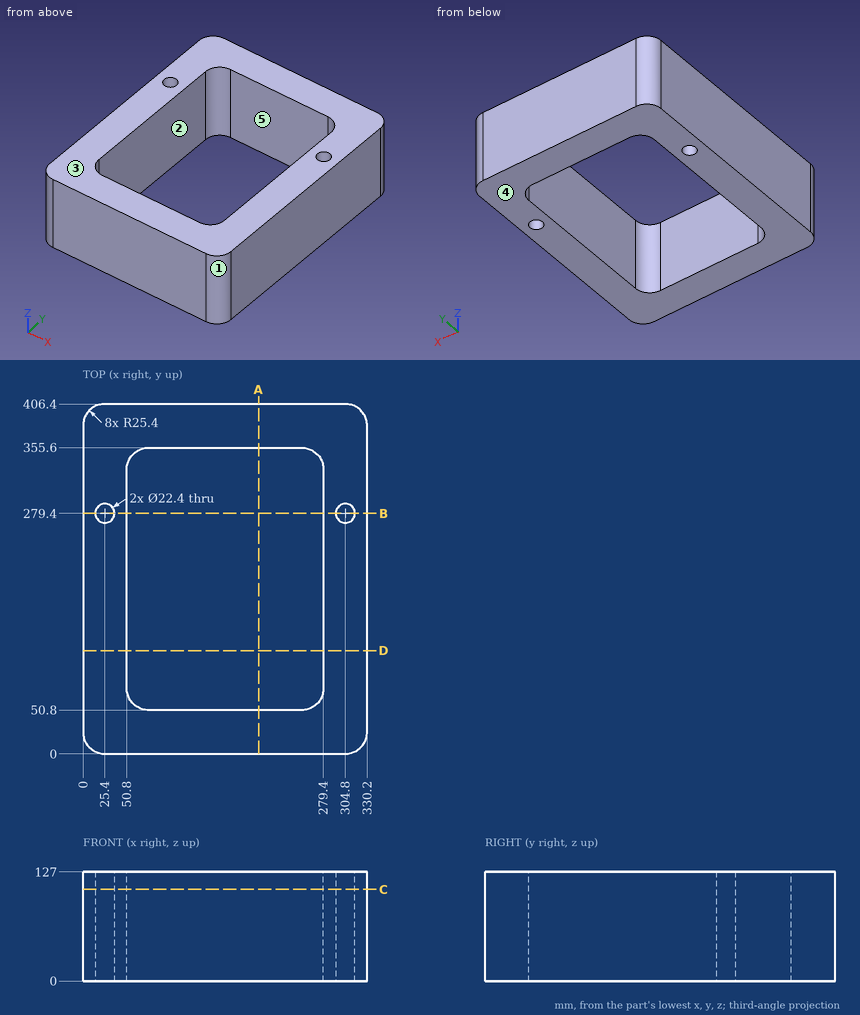
Geometry: see drawing. Coordinates: mm, zero at the bounding-box minimum. A direction names the side the tool comes from. Give positions to 0.01 mm unless a question says otherwise; leave off trailing zeros. Loops run counter-clockwise (first coordinate to the right, second up) from the corner with the lowest first, then second, coordinate; pieces in that order, holes last. Notation, with made-up numbers: (68.25, 50.25) -> (121.25, 50.25) arc R17 ccw to (121.25, 78.25) -> close; hole circle Ø9 at (81.25, -39). An arc over 180 degrees is marked (long way). Use one line per item in the form item = value.
Item 1: Section query D-D on y = 120. Output: boundary loops of the cut face in (x, z).
A:
outline = (0, 0) -> (50.8, 0) -> (50.8, 127) -> (0, 127) -> close; (279.4, 0) -> (330.2, 0) -> (330.2, 127) -> (279.4, 127) -> close
Item 2: Pin query (flat end, axial travel): P1, Ø2, axis at x = 222, z = 35, coming from the -Y side. Return the tip coordinate at first contact, or that it passes through.
A:
P1 = 0
Item 3: Access query for the marked faces 4 and 5. Directions: +Z, -Z, +X, -X, +Y, -Y. A direction counts if a zero-diameter tool reaches every point of the face in a straight line with its end or side. Return the directions, or none.
A:
face_4 = -Z, +X, -X, +Y, -Y
face_5 = +Z, -Z
Item 4: Section query B-B on y = 279.4. Output: boundary loops of the cut face in (x, z), and give its area (3 significant figures).
A:
outline = (0, 0) -> (14.2, 0) -> (14.2, 127) -> (0, 127) -> close; (36.6, 0) -> (50.8, 0) -> (50.8, 127) -> (36.6, 127) -> close; (279.4, 0) -> (293.6, 0) -> (293.6, 127) -> (279.4, 127) -> close; (316, 0) -> (330.2, 0) -> (330.2, 127) -> (316, 127) -> close
area = 7,210 mm^2
Item 5: Draft query along Y for the marked faces 1, 2 and 3. Return one class per face: pulls with the +Y half, pulls with the -Y half, needs draft (parallel to the pull), parting line crosses it, or undercut.
A:
face_1 = pulls with the -Y half
face_2 = undercut
face_3 = needs draft
Item 6: Section query A-A on x = 204. Output: boundary loops of the cut face in (y, z).
A:
outline = (0, 0) -> (50.8, 0) -> (50.8, 127) -> (0, 127) -> close; (355.6, 0) -> (406.4, 0) -> (406.4, 127) -> (355.6, 127) -> close
Item 7: Line query: probe 1 along X at (y, z) = (279, 65); probe 2 along Y at (x, z) = (304.8, 33); probe 3 along X at (y, z) = (78.5, 78.5). Output: solid intervals per line, ascending.
A:
probe_1 = 0 to 14.21, 36.59 to 50.8, 279.4 to 293.61, 315.99 to 330.2
probe_2 = 0 to 268.2, 290.6 to 406.4
probe_3 = 0 to 50.8, 279.4 to 330.2
Item 8: Section query C-C on z = 106.5. Output: boundary loops of the cut face in (x, y).
A:
outline = (0, 25.4) arc R25.4 ccw to (25.4, 0) -> (304.8, 0) arc R25.4 ccw to (330.2, 25.4) -> (330.2, 381) arc R25.4 ccw to (304.8, 406.4) -> (25.4, 406.4) arc R25.4 ccw to (0, 381) -> close; hole circle Ø22.4 at (25.4, 279.4); hole (50.8, 76.2) arc R25.4 ccw to (76.2, 50.8) -> (254, 50.8) arc R25.4 ccw to (279.4, 76.2) -> (279.4, 330.2) arc R25.4 ccw to (254, 355.6) -> (76.2, 355.6) arc R25.4 ccw to (50.8, 330.2) -> close; hole circle Ø22.4 at (304.8, 279.4)
